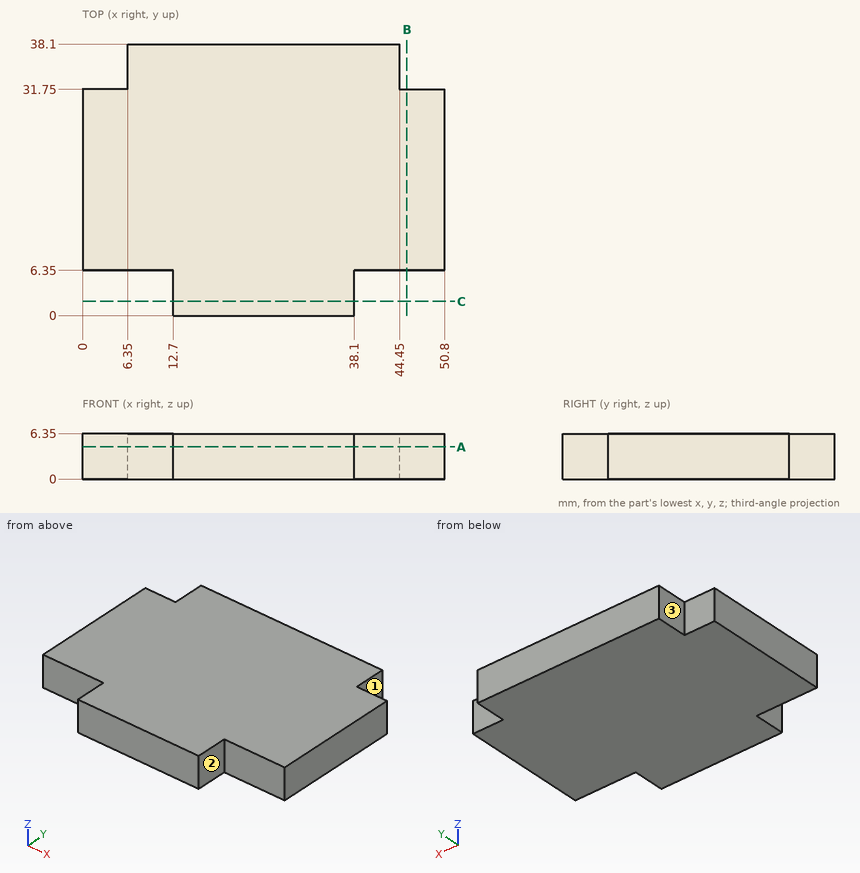
Study the drawing (mm; zero at the part's minimum x, y, z) and answer. A direction names the side the tool comes from. Round coordinates to 2 decimals unless told otherwise and drop trailing zeros. Write each loop counter-clockwise with the first axis right and the second up, starting at its lowest first coordinate (ties: lowest second). Pieces come first, ordered by that corner, then holes. Notation, with made-up numbers: (25.5, -36) -> (69.5, -36) arc R24 ccw to (69.5, -17) -> close; hole circle Ø2 at (-25.5, 84.5). An arc over 180 degrees is marked (long way). Write item = value, one per line.
1) Section B-B on x = 45.5 is taken. Write down the section's boundary in (y, z), plus the area to 3 significant figures.
Check values:
outline = (6.35, 0) -> (31.75, 0) -> (31.75, 6.35) -> (6.35, 6.35) -> close
area = 161 mm²
2) Which of the six approach directions +Z, -Z, +X, -X, +Y, -Y give full straight-line access (tool end or side, diameter ignored) to the marked faces 1, 2 and 3?
Check values:
face_1 = +Z, -Z, +X, +Y
face_2 = +Z, -Z, +X, -Y
face_3 = +Z, -Z, -X, +Y
3) Given pin 1 (3 mm diameter, centred on y = 2, z = 2.5, fed in from -X); pin 2 (3 mm diameter, centred on x = 43, z = 4, fed in from -Y); pin 3 (3 mm diameter, centred on y = 35, z = 3.5, fed in from -X), each flat-ended and moving along its own axis, determine where each tip first touches the part or whether it passes through.
Check values:
pin_1 = 12.7
pin_2 = 6.35
pin_3 = 6.35
4) Straight lines are drawn through the part: line 1 along X through (y, z) = (35.5, 4); line 2 along Y through (x, z) = (41, 3.5); line 3 along Y through (x, z) = (46.5, 2.5). For each, find the intervals that lie inside material, in ascending order. Write a range as [from, to].
Check values:
line_1 = [6.35, 44.45]
line_2 = [6.35, 38.1]
line_3 = [6.35, 31.75]
5) Section C-C on y = 2 is taken. Write down the section's boundary in (x, z), plus the area to 3 significant figures.
Check values:
outline = (12.7, 0) -> (38.1, 0) -> (38.1, 6.35) -> (12.7, 6.35) -> close
area = 161 mm²
6) Section A-A on z = 4.5 is taken. Write down the section's boundary in (x, y), plus the area to 3 significant figures.
Check values:
outline = (0, 6.35) -> (12.7, 6.35) -> (12.7, 0) -> (38.1, 0) -> (38.1, 6.35) -> (50.8, 6.35) -> (50.8, 31.75) -> (44.45, 31.75) -> (44.45, 38.1) -> (6.35, 38.1) -> (6.35, 31.75) -> (0, 31.75) -> close
area = 1,690 mm²
